CAD build for the part. Positions are in the model's coordinates, mm. Give positions to 0.01 mm unless a question says otherwise; leave off trailing zeros. Order: outer loops, then holes, each group sorted by start corner. A loop starts at its lowest first (then second) coordinate and runs counter-clockwise, first axis right, second up. Notation, with made-up numbers: (78, 60) -> (92, 60) arc R27 ccw to (92, 97) -> close; hole circle Ø7 at (-20.75, 76). An arc over 180 degrees is marked (long way). Use one line per item in the form item = value. Start each with the question number.
1) Cut at B-B, the plane z = 18.5. Give the cut face in (x, y).
2) Probe line 1 (Y direction, x = -128, z = 18.75); line 2 (X direction, y = 27.75, z = 22.25); line 3 (Y direction, x = -129, z = 18.75). List the from-to ranges inside material, lowest first.
3) Mould opens along Y. For faces 1 (the face through (-125.274, 29.176, 21.006)), 2 (the face through (-127, 26, 17.46)), 3 (the face through (-120.982, 30.527, 23.906)) say: pulls with the +Y half, pulls with the -Y half, needs draft (parallel to the pull), parting line crosses it, or undercut.
4) Cut at A-A, the plane z = 21.75. Give the cut face in (x, y).
5) Drop a flat-ended pin along its axis: P1, Ø1.5, axis at x = -130, z = 22, coming from the -Y side. Give the stop position or say it passes through.
from build123d import *


with BuildPart() as part:
    # Sketch1 → Revolve1 (revolve)
    with BuildSketch(Plane(origin=(0, 28.574866342, 0), x_dir=(1, 0, 0), z_dir=(0, 1, 0))):
        with BuildLine():
            Line((-120.681601968, -17.71), (-120.931601968, -17.46))
            Line((-120.931601968, -17.46), (-124.931601968, -17.46))
            Line((-124.931601968, -17.46), (-125.181601968, -17.71))
            Line((-125.181601968, -17.71), (-125.181601968, -24.21))
            Line((-125.181601968, -24.21), (-124.931601968, -24.46))
            Line((-124.931601968, -24.46), (-120.931601968, -24.46))
            Line((-120.931601968, -24.46), (-120.681601968, -24.21))
            Line((-120.681601968, -24.21), (-120.681601968, -23.61))
            ThreePointArc((-120.681601968, -23.61), (-122.681601968, -20.96), (-120.681601968, -18.31))
            Line((-120.681601968, -18.31), (-120.681601968, -17.71))
        make_face()
    revolve(axis=Axis((-127.181601968, 28.574866342, 17.46), (0, 0, 1)))


solid = part.part
Result:
q1.outline = circle Ø12.03 at (-127.18, 28.57); hole circle Ø4 at (-127.18, 28.57)
q2.line_1 = 23.03 to 26.75, 30.4 to 34.12
q2.line_2 = -131.93 to -129, -125.36 to -122.43
q2.line_3 = 23.27 to 27.74, 29.41 to 33.88
q3.face_1 = undercut
q3.face_2 = needs draft
q3.face_3 = parting line crosses it
q4.outline = circle Ø9.23 at (-127.18, 28.57); hole circle Ø4 at (-127.18, 28.57)
q5.P1 = 24.12
